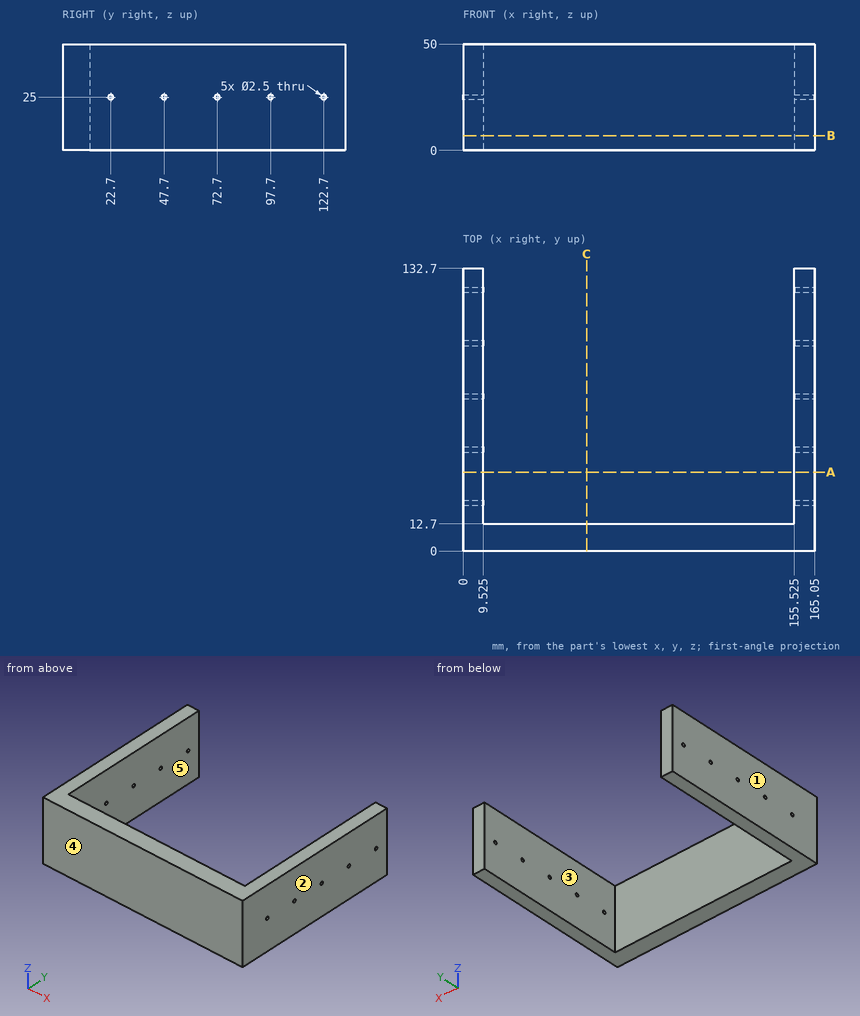
Answer from the drawing. Dimensions are ordinates in mm from the lowest x, y and z of the part. A direction names the side the tool comes from. Coordinates: 2 decimals unless noted, no trailing zeros. Loops run counter-clockwise (first coordinate to the right, second up) from the corner with the lowest first, then second, coordinate; pieces in that order, holes last.
Q1. The part is cut by section C-C on x = 58. Write down the section's boundary in (y, z).
Q2. The part is cut by section B-B on z = 7. Write down the section's boundary in (x, y) (3 decimals).
Q3. Which of the six approach directions +Z, -Z, +X, -X, +Y, -Y give full straight-line access (tool end or side, diameter ignored) to the marked faces 4 and 5?
Q4. Consider probe 1 along Y at (x, z) = (159.25, 25); probe 2 along X at (y, z) = (38.5, 8.5) (3 decimals); probe 3 along Z at (x, y) = (159.5, 97.7). Determine where each line is inside the solid, lowest interval first.
Q5. The mould has two halves that part along X. Classify the marked faces 1, 2 and 3: +X half, -X half, draft (parallel to the pull), parting line (faces both ways), or undercut.
Q6. The part is cut by section A-A on y = 37. Write down the section's boundary in (x, z) (3 decimals).
Results below:
1. outline: (0, 0) - (12.7, 0) - (12.7, 50) - (0, 50) - close
2. outline: (0, 0) - (165.05, 0) - (165.05, 132.7) - (155.525, 132.7) - (155.525, 12.7) - (9.525, 12.7) - (9.525, 132.7) - (0, 132.7) - close
3. face 4: +Z, -Z, +X, -X, -Y
3. face 5: +Z, -Z, +Y
4. probe 1: y = 0 to 21.45, 23.95 to 46.45, 48.95 to 71.45, 73.95 to 96.45, 98.95 to 121.45, 123.95 to 132.7
4. probe 2: x = 0 to 9.525, 155.525 to 165.05
4. probe 3: z = 0 to 23.75, 26.25 to 50
5. face 1: -X half
5. face 2: +X half
5. face 3: undercut
6. outline: (0, 0) - (9.525, 0) - (9.525, 50) - (0, 50) - close; (155.525, 0) - (165.05, 0) - (165.05, 50) - (155.525, 50) - close
